```python
from build123d import *

# Parameters (mm, degrees)
F1_DEPTH = 12.5
F2_SIZE  = 5


with BuildPart() as f1:
    # F0 (on Front) → F1 (new body, symmetric)
    with BuildSketch(Plane.XZ):
        with BuildLine():
            Line((0, 62.005542), (0, 0))
            Line((0, 0), (33.04759, 0))
            Line((33.04759, 0), (33.04759, 62.005542))
            ThreePointArc((33.04759, 62.005542), (16.523795, 78.529337), (0, 62.005542))
        make_face()
    extrude(amount=F1_DEPTH, both=True)

    # F2
    f2_edges = [f1.edges().sort_by_distance(p)[0] for p in [
        (16.523795, -12.5, 78.529337),
        (16.523795, 12.5, 78.529337),
    ]]
    chamfer(f2_edges, length=F2_SIZE)


solid = f1.part
```
Verification items for the finished model (mm, model axes). Coordinates: 2 decimals unless noted, no trailing zeros. Order: outer loops, then holes, each group sorted by start corner. A loop starts at its lowest first (then second) coordinate and runs counter-clockwise, first axis right, second up. Notation, with made-up numbers: (-26.5, 26.5) - (-20.5, 26.5) arc R12 ccw to (-20.5, 45.5) - close; hole circle Ø9 at (13.5, 52). An arc over 180 degrees is marked (long way). Return JSON: item names as keys, results as strings.
(1) Section check C-C, the plane y = 8.25. Record the cut outline in (x, z), and give its area (3 significant figures).
Filled sheet:
{"outline": "(0.75, 0) - (32.3, 0) - (32.3, 62.01) arc R15.77 ccw to (0.75, 62.01) - close", "area": "2,350 mm^2"}
(2) Section check B-B, the plane y = -6.75. Record the cut outline in (x, z).
Filled sheet:
{"outline": "(0, 0) - (33.05, 0) - (33.05, 62.01) arc R16.52 ccw to (0, 62.01) - close"}
(3) Section check A-A, the plane z = 25. Record the cut outline in (x, y).
Filled sheet:
{"outline": "(0, -7.5) - (5, -12.5) - (28.05, -12.5) - (33.05, -7.5) - (33.05, 7.5) - (28.05, 12.5) - (5, 12.5) - (0, 7.5) - close"}
(4) Go/stop test with flat-tipped pins: pin 1 (1.5 mm diameter, centred on y = -1.5, z = 67, fed in from +X); pin 2 (6 mm diameter, centred on x = 25.5, y = -1, fed in from -Z); pin 3 (4 mm diameter, centred on x = 22.5, y = -4, fed in from +Z); pin 4 (1.5 mm diameter, centred on x = 4, y = -8.5, fed in from +Z). Record where each tip stops, or that it passes through.
Filled sheet:
{"pin 1": "stops at x = 32.49", "pin 2": "stops at z = 0", "pin 3": "stops at z = 78.04", "pin 4": "stops at z = 72.69"}
(5) Thickness scan on line 1 along Z through (x, y) = (16.5, 3.75); line 2 along Z through (x, y) = (4, 6.5); line 3 along Y through (x, z) = (4.5, 48). Record the ranges inside material, lowest first.
Filled sheet:
{"line 1": "z = 0 to 78.53", "line 2": "z = 0 to 72.78", "line 3": "y = -12 to 12"}
(6) Mould release check, pull along Y, two halves, no side actions. Record for faces 1 (the flat face through (33.048, 0, 31)), 2 (the flat face through (2.5, -10, 31.4)), 3 (the flat face through (2.5, 10, 31.4)): pulls with the +Y half, pulls with the -Y half, needs draft (parallel to the pull), parting line crosses it, or undercut.
Filled sheet:
{"face 1": "needs draft", "face 2": "pulls with the -Y half", "face 3": "pulls with the +Y half"}
